Work out the finished part from the listing and answer in its coordinate system (mm). A direction names the side the tool comes from. Round coordinates to 2 decimals unless told otherwise and drop trailing zeros. Write each loop counter-clockwise with the first axis right and the second up, starting at its lowest first coordinate (ties: lowest second). Pieces come first, ordered by that corner, then holes. Notation, with made-up numbers: (31.5, 58) - (56.5, 58) arc R18 ccw to (56.5, 62) - close; hole circle Ø4 at (-13, 26). An arc over 180 degrees is marked (long way). Answer as a JSON object with one key per item and string values.
```python
from build123d import *

# Parameters (mm, degrees)
MODEL_R             = 1.5
BOSS_EXTRUDE1_DEPTH = 6.6


with BuildPart() as part:
    # Model → Boss-Extrude1 (new body)
    with BuildSketch(Plane.XY):
        with BuildLine():
            Line((12.114213562, 5.985786438), (-6.714213562, 24.814213562))
            ThreePointArc((-6.714213562, 24.814213562), (-7.36306026, 25.247759065), (-8.128427125, 25.4))
            Line((-8.128427125, 25.4), (-10.7, 25.4))
            ThreePointArc((-10.7, 25.4), (-12.114213562, 24.814213562), (-12.7, 23.4))
            Line((-12.7, 23.4), (-12.7, 17.257211543))
            ThreePointArc((-12.7, 17.257211543), (-12.355939499, 16.135666013), (-11.442135624, 15.4))
            Line((-11.442135624, 15.4), (2.7, 1.257864376))
            Line((2.7, 1.257864376), (2.7, -1.257864376))
            Line((2.7, -1.257864376), (-11.442135624, -15.4))
            ThreePointArc((-11.442135624, -15.4), (-12.355939499, -16.135666013), (-12.7, -17.257211543))
            Line((-12.7, -17.257211543), (-12.7, -23.4))
            ThreePointArc((-12.7, -23.4), (-12.114213562, -24.814213562), (-10.7, -25.4))
            Line((-10.7, -25.4), (-8.128427125, -25.4))
            ThreePointArc((-8.128427125, -25.4), (-7.36306026, -25.247759065), (-6.714213562, -24.814213562))
            Line((-6.714213562, -24.814213562), (12.114213562, -5.985786438))
            ThreePointArc((12.114213562, -5.985786438), (12.547759065, -5.33693974), (12.7, -4.571572875))
            Line((12.7, -4.571572875), (12.7, 4.571572875))
            ThreePointArc((12.7, 4.571572875), (12.547759065, 5.33693974), (12.114213562, 5.985786438))
        make_face()
        with Locations((-9.414213562, 20.4)):
            Circle(MODEL_R, mode=Mode.SUBTRACT)
        with Locations((-9.414213562, -20.4)):
            Circle(MODEL_R, mode=Mode.SUBTRACT)
    extrude(amount=BOSS_EXTRUDE1_DEPTH)


solid = part.part
```
Item 1: A cutting plane is placed at A-A (y = -20.4). Write down the section's boundary in (x, z).
Results found:
{"outline": "(-12.7, 0) - (-10.91, 0) - (-10.91, 6.6) - (-12.7, 6.6) - close; (-7.91, 0) - (-2.3, 0) - (-2.3, 6.6) - (-7.91, 6.6) - close"}
Item 2: For faces 1 (the flat face through (2.7, 0, 3)), 2 (the flat face through (2.6, -15.5, 3.3)), determine the directions among +Z, -Z, +X, -X, +Y, -Y from which every point of the face is accessible in a straight line to the end or side of a thin tool.
Results found:
{"face 1": "+Z, -Z, -X", "face 2": "+Z, -Z, +X, -Y"}
Item 3: Consider line 1 along Y through (x, z) = (-10.25, 3.25); line 2 along Y through (x, z) = (-9, 4); line 3 along X through (y, z) = (0, 2). Determine where each line is inside the solid, lowest interval first.
Results found:
{"line 1": "-25.4 to -21.65, -19.15 to -14.21, 14.21 to 19.15, 21.65 to 25.4", "line 2": "-25.4 to -21.84, -18.96 to -12.96, 12.96 to 18.96, 21.84 to 25.4", "line 3": "2.7 to 12.7"}
Item 4: A cutting plane is placed at C-C (x = 1). Write down the section's boundary in (y, z), and give its area (3 significant figures).
Results found:
{"outline": "(-17.1, 0) - (-2.96, 0) - (-2.96, 6.6) - (-17.1, 6.6) - close; (2.96, 0) - (17.1, 0) - (17.1, 6.6) - (2.96, 6.6) - close", "area": "187 mm²"}
Item 5: A cutting plane is placed at B-B (z = 2.25). Write down the section's boundary in (x, y).
Results found:
{"outline": "(-12.7, -23.4) arc R2 ccw to (-10.7, -25.4) - (-8.13, -25.4) arc R2 ccw to (-6.71, -24.81) - (12.11, -5.99) arc R2 ccw to (12.7, -4.57) - (12.7, 4.57) arc R2 ccw to (12.11, 5.99) - (-6.71, 24.81) arc R2 ccw to (-8.13, 25.4) - (-10.7, 25.4) arc R2 ccw to (-12.7, 23.4) - (-12.7, 17.26) arc R2 ccw to (-11.44, 15.4) - (2.7, 1.26) - (2.7, -1.26) - (-11.44, -15.4) arc R2 ccw to (-12.7, -17.26) - close; hole circle Ø3 at (-9.41, -20.4); hole circle Ø3 at (-9.41, 20.4)"}
Item 6: Each of these flat-tipped pins is pushed along its axis until it touches: P1, Ø1, axis at y = 14.5, z = 1.5, coming from the -X side; P2, Ø3, axis at y = 10.5, z = 1.5, coming from the +X side; P3, Ø1.5, axis at x = 10, z = 4.5, coming from the +Y side; P4, Ø1.5, axis at x = 0, y = 17, coming from the -Z side. Where does it stop, or does it pass through?
Results found:
{"P1": "x = -11.04", "P2": "x = 9.1", "P3": "y = 8.85", "P4": "z = 0"}
Item 7: Determine the mould class of faces 3 (the flat face through (-4.47, 8.43, 3.25)), 4 (the cylindrical face through (-8.608, -19.135, 3.254)), 5 (the cylindrical face through (-7.353, 25.244, 3.254)) for opening direction X: pulls with the +X half, pulls with the -X half, needs draft (parallel to the pull), parting line crosses it, or undercut.
Results found:
{"face 3": "pulls with the -X half", "face 4": "undercut", "face 5": "pulls with the +X half"}
Item 8: A cutting plane is placed at D-D (x = -9). Write down the section's boundary in (y, z), and give its area (3 significant figures).
Results found:
{"outline": "(-25.4, 0) - (-21.84, 0) - (-21.84, 6.6) - (-25.4, 6.6) - close; (-18.96, 0) - (-12.96, 0) - (-12.96, 6.6) - (-18.96, 6.6) - close; (12.96, 0) - (18.96, 0) - (18.96, 6.6) - (12.96, 6.6) - close; (21.84, 0) - (25.4, 0) - (25.4, 6.6) - (21.84, 6.6) - close", "area": "126 mm²"}
